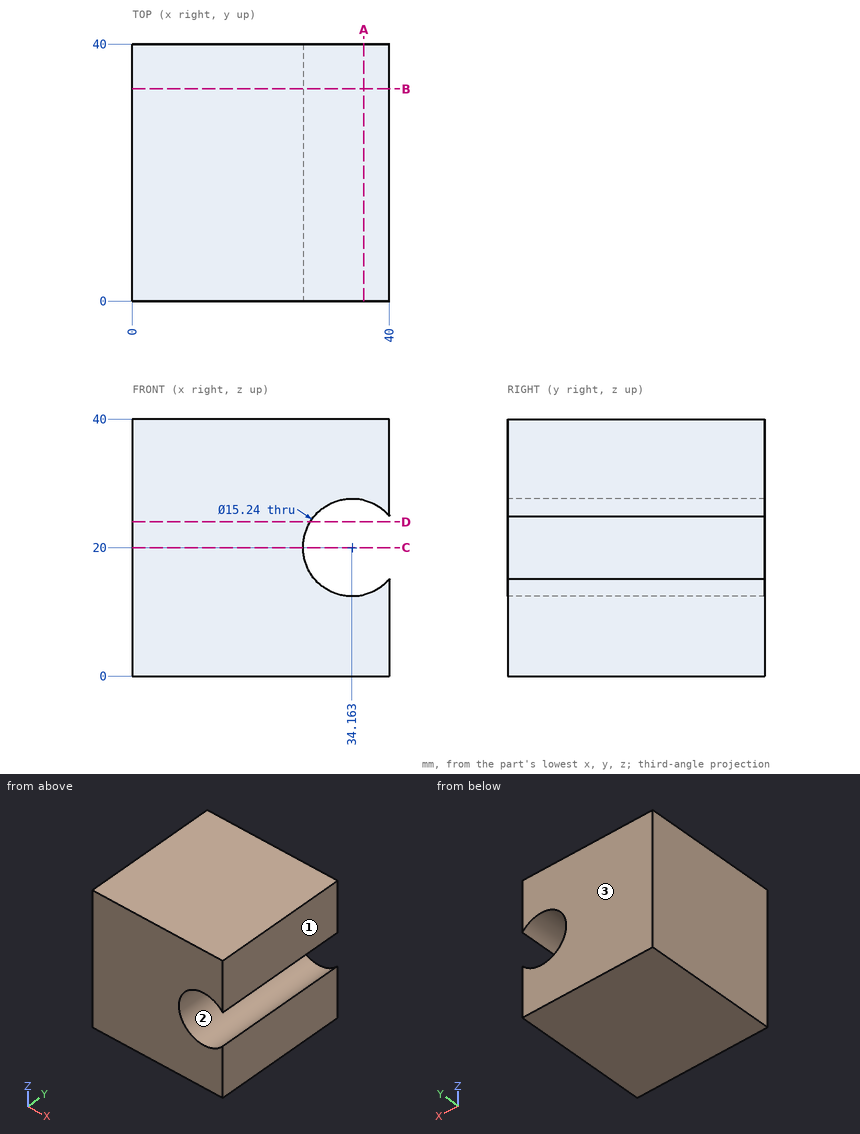
Input: dimensioned drawing with shaded views. Units: mm. Origin: part minimum x, y, z. Round coordinates to 2 decimals unless told otherwise and drop trailing zeros. Order: outer loops, then holes, each group sorted by start corner. A loop starts at its lowest first (then second) coordinate and runs counter-clockwise, first axis right, second up. Notation, with made-up numbers: (-28.5, 78.5) -> (-7.5, 78.5) arc R31 cw to (-7.5, 109.5) -> close; hole circle Ø6 at (-31, 74.25). An arc over 180 degrees is marked (long way). One line per item, written item: value. Start each with the question number.
Q1. Section query D-D (z = 24). Return the cut outline in (x, y).
Q2. Section query A-A (x = 36). Return the cut outline in (y, z) (1 decimal).
Q3. Section query C-C (z = 20). Return the cut outline in (x, y), plus the area to 3 significant figures.
Q4. Section query B-B (y = 33). Return the cut outline in (x, z).
Q5. Draft query along X for the marked faces 1, 2 and 3. Return one class per face: pulls with the +X half, pulls with the -X half, needs draft (parallel to the pull), parting line crosses it, or undercut.
Q6. Material intervals for probe 1 along Z at (x, y) = (34.5, 27); probe 2 along X at (y, z) = (37, 20); probe 3 along Z at (x, y) = (29.5, 34.5) (1 decimal), sorted ascending.
Findings below:
1. outline: (0, 0) -> (27.68, 0) -> (27.68, 40) -> (0, 40) -> close
2. outline: (0, 0) -> (40, 0) -> (40, 12.6) -> (0, 12.6) -> close; (0, 27.4) -> (40, 27.4) -> (40, 40) -> (0, 40) -> close
3. outline: (0, 0) -> (26.54, 0) -> (26.54, 40) -> (0, 40) -> close
3. area: 1,060 mm²
4. outline: (0, 0) -> (40, 0) -> (40, 15.1) arc R7.62 cw (long way) to (40, 24.9) -> (40, 40) -> (0, 40) -> close
5. face 1: pulls with the +X half
5. face 2: undercut
5. face 3: needs draft
6. probe 1: 0 to 12.39, 27.61 to 40
6. probe 2: 0 to 26.54
6. probe 3: 0 to 14, 26 to 40
